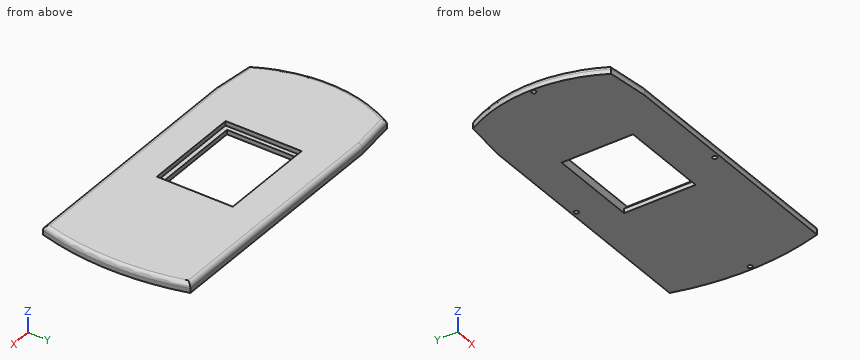
from build123d import *

# Parameters (mm, degrees)
EXTRU_MINCE1_DEPTH      = 10
ESQUISSE1_25_W          = 40
ESQUISSE1_25_H          = 136
ESQUISSE1_25_W_2        = 20
ESQUISSE1_25_H_2        = 2
ESQUISSE1_25_R          = 2.5
BOSS_EXTRU_3_DEPTH      = 10
ESQUISSE1_26_R          = 2.5
ENL_V_MAT_EXTRU_1_DEPTH = 5
ESQUISSE1_27_R          = 2.5
ENL_V_MAT_EXTRU_2_DEPTH = 5
ESQUISSE1_28_R          = 2.5
ENL_V_MAT_EXTRU_3_DEPTH = 5
ESQUISSE1_29_R          = 2.5
ENL_V_MAT_EXTRU_4_DEPTH = 5
CONG_5_R                = 5
BOSS_EXTRU_4_DEPTH      = 5


with BuildPart() as part:
    # Esquisse1 → Extru.-Mince1 (new body)
    with BuildSketch(Plane.XY):
        with BuildLine():
            Line((-199.071776485, 47.699787448), (-153.336718001, 52.844981528))
            Line((-153.336718001, 52.844981528), (122.846559315, 52.844981528))
            ThreePointArc((122.846559315, 52.844981528), (134.520037722, -29.655018472), (122.846559315, -112.155018472))
            Line((122.846559315, -112.155018472), (-153.336718001, -112.155018472))
            Line((-153.336718001, -112.155018472), (-199.071776485, -107.009824393))
            ThreePointArc((-199.071776485, -107.009824393), (-219.440219924, -29.655018472), (-199.071776485, 47.699787448))
        make_face()
        with BuildLine():
            Line((-192.775986612, 38.344981528), (-152.775986612, 42.844981528))
            Line((-152.775986612, 42.844981528), (115.224013388, 42.844981528))
            ThreePointArc((115.224013388, 42.844981528), (124.520037722, -29.655018472), (115.224013388, -102.155018472))
            Line((115.224013388, -102.155018472), (-152.775986612, -102.155018472))
            Line((-152.775986612, -102.155018472), (-192.775986612, -97.655018472))
            ThreePointArc((-192.775986612, -97.655018472), (-209.440219924, -29.655018472), (-192.775986612, 38.344981528))
        make_face(mode=Mode.SUBTRACT)
    extrude(amount=EXTRU_MINCE1_DEPTH)

    # Esquisse1_25 → Boss.-Extru.3 (add)
    # profile 1 of 14: a face of its own
    with BuildSketch(Plane.XY):
        Polygon((-192.775986612, 42.844981528), (-192.775986612, 38.344981528), (-152.775986612, 42.844981528), align=None)
    # profile 2 of 14: a face of its own
    with BuildSketch(Plane.XY):
        with Locations((-172.775986612, -29.655018472)):
            Rectangle(ESQUISSE1_25_W, ESQUISSE1_25_H)
    # profile 3 of 14: a face of its own
    with BuildSketch(Plane.XY):
        Polygon((-152.775986612, 42.844981528), (-192.775986612, 38.344981528), (-152.775986612, 38.344981528), align=None)
    # profile 4 of 14: a face of its own
    with BuildSketch(Plane.XY):
        with BuildLine():
            Line((-192.775986612, -97.655018472), (-192.775986612, 38.344981528))
            ThreePointArc((-192.775986612, 38.344981528), (-209.440219924, -29.655018472), (-192.775986612, -97.655018472))
        make_face()
    # profile 5 of 14: a face of its own
    with BuildSketch(Plane.XY):
        Polygon((-144.987389646, 42.844981528), (-152.775986612, 42.844981528), (-152.775986612, 38.344981528), (-152.775986612, -97.655018472), (-152.775986612, -102.155018472), (-144.987389646, -102.155018472), (-144.987389646, -100.155018472), (-124.987389646, -100.155018472), (-124.987389646, -102.155018472), (115.224013388, -102.155018472), (115.224013388, 42.844981528), (-124.987389646, 42.844981528), (-124.987389646, 40.844981528), (-144.987389646, 40.844981528), align=None)
        Polygon((-112.169243918, 12.844981528), (-107.169243918, 12.844981528), (-7.169243918, 12.844981528), (-2.169243918, 12.844981528), (-2.169243918, -72.155018472), (-112.169243918, -72.155018472), align=None, mode=Mode.SUBTRACT)
    # profile 6 of 14: a face of its own
    with BuildSketch(Plane.XY):
        Polygon((-152.775986612, -102.155018472), (-192.775986612, -97.655018472), (-192.775986612, -102.155018472), align=None)
    # profile 7 of 14: a face of its own
    with BuildSketch(Plane.XY):
        Polygon((-152.775986612, -97.655018472), (-192.775986612, -97.655018472), (-152.775986612, -102.155018472), align=None)
    # profile 8 of 14: a face of its own
    with BuildSketch(Plane.XY):
        with Locations((-134.987389646, 41.844981528)):
            Rectangle(ESQUISSE1_25_W_2, ESQUISSE1_25_H_2)
    # profile 9 of 14: a face of its own
    with BuildSketch(Plane.XY):
        with Locations((-134.987389646, -101.155018472)):
            Rectangle(ESQUISSE1_25_W_2, ESQUISSE1_25_H_2)
    # profile 10 of 14: a face of its own
    with BuildSketch(Plane.XY):
        with BuildLine():
            ThreePointArc((115.224013388, -102.155018472), (124.520037722, -29.655018472), (115.224013388, 42.844981528))
            Line((115.224013388, 42.844981528), (115.224013388, -102.155018472))
        make_face()
    # profile 11 of 14: a face of its own
    with BuildSketch(Plane.XY):
        with Locations((-215.775986612, -32.155018472)):
            Circle(ESQUISSE1_25_R)
    # profile 12 of 14: a face of its own
    with BuildSketch(Plane.XY):
        with Locations((130.224013388, -32.155018472)):
            Circle(ESQUISSE1_25_R)
    # profile 13 of 14: a face of its own
    with BuildSketch(Plane.XY):
        with Locations((-33.549027095, -107.155018472)):
            Circle(ESQUISSE1_25_R)
    # profile 14 of 14: a face of its own
    with BuildSketch(Plane.XY):
        with Locations((-33.549027095, 47.844981528)):
            Circle(ESQUISSE1_25_R)
    extrude(amount=BOSS_EXTRU_3_DEPTH)

    # Esquisse1_26 → Enl_v. mat.-Extru.1 (cut)
    with BuildSketch(Plane.XY):
        with Locations((130.224013388, -32.155018472)):
            Circle(ESQUISSE1_26_R)
    extrude(amount=ENL_V_MAT_EXTRU_1_DEPTH, mode=Mode.SUBTRACT)

    # Esquisse1_27 → Enl_v. mat.-Extru.2 (cut)
    with BuildSketch(Plane.XY):
        with Locations((-33.549027095, -107.155018472)):
            Circle(ESQUISSE1_27_R)
    extrude(amount=ENL_V_MAT_EXTRU_2_DEPTH, mode=Mode.SUBTRACT)

    # Esquisse1_28 → Enl_v. mat.-Extru.3 (cut)
    with BuildSketch(Plane.XY):
        with Locations((-33.549027095, 47.844981528)):
            Circle(ESQUISSE1_28_R)
    extrude(amount=ENL_V_MAT_EXTRU_3_DEPTH, mode=Mode.SUBTRACT)

    # Esquisse1_29 → Enl_v. mat.-Extru.4 (cut)
    with BuildSketch(Plane.XY):
        with Locations((-215.775986612, -32.155018472)):
            Circle(ESQUISSE1_29_R)
    extrude(amount=ENL_V_MAT_EXTRU_4_DEPTH, mode=Mode.SUBTRACT)

    # Cong_5
    cong_5_edges = [part.edges().sort_by_distance(p)[0] for p in [
        (134.520037722, -29.655018472, 10),
        (-15.245079343, 52.844981528, 10),
        (-176.204247243, 50.272384488, 10),
        (-219.440219924, -29.655018472, 10),
        (-176.204247243, -109.582421433, 10),
        (-15.245079343, -112.155018472, 10),
    ]]
    fillet(cong_5_edges, radius=CONG_5_R)

    # Esquisse1_30 → Boss.-Extru.4 (add)
    with BuildSketch(Plane.XY):
        Polygon((-7.169243918, -67.155018472), (-107.169243918, -67.155018472), (-107.169243918, 12.844981528), (-112.169243918, 12.844981528), (-112.169243918, -72.155018472), (-2.169243918, -72.155018472), (-2.169243918, 12.844981528), (-7.169243918, 12.844981528), align=None)
    extrude(amount=BOSS_EXTRU_4_DEPTH)


solid = part.part
Can you work these out from the model? Positions are in its coordinate system, mm. Round coordinates to 2 decimals unless told otherwise and drop trailing zeros. Write each loop counter-clockwise with the first axis right and the second up, starting at its lowest first coordinate (ties: lowest second). Pieces come first, ordered by that corner, then holes. Notation, with made-up numbers: M 73.25,88 L 132.25,88 A6 cw 132.25,97 Z; hole C 75,-2 d9. An arc over 180 degrees is marked long. Use a Markdown table: item, result.
Item 1: I want a section at A-A (x = -99.5). List the corners of the cut face in (y, z) for me, and give its area (3 significant figures).
Found:
| item | result |
|---|---|
| outline | M -112.16,0 L -67.16,0 L -67.16,5 L -72.16,5 L -72.16,10 L -107.16,10 A5 ccw -112.16,5 Z; M 12.84,0 L 52.84,0 L 52.84,5 A5 ccw 47.84,10 L 12.84,10 Z |
| area | 814 mm2 |
Item 2: If I drill on line 1 along Y through (x, z) = (-45, 4.25); line 2 along X through (y, z) = (-45.5, 8.75); line 3 along Y through (x, z) = (-101.5, 7.75), over which ranges is the centre line in solid material (lowest first)? Write a range as [from, to].
Found:
| item | result |
|---|---|
| line 1 | y = [-112.16, -67.16], [12.84, 52.84] |
| line 2 | x = [-216.94, -112.17], [-2.17, 132.4] |
| line 3 | y = [-111.33, -72.16], [12.84, 52.02] |
Item 3: I want a section at B-B (z = 6.75). List the corners of the cut face in (x, y) for me, and give its area (3 significant figures).
Found:
| item | result |
|---|---|
| outline | M -198.88,-106.71 L -153.32,-111.84 L 122.61,-111.84 A297.05 ccw 122.61,52.53 L -153.32,52.53 L -198.88,47.4 A156.76 ccw Z; hole M -112.17,-72.16 L -2.17,-72.16 L -2.17,12.84 L -112.17,12.84 Z |
| area | 46,600 mm2 |
Item 4: For pin 1 Ø1.5 at (x, y) = (-214.5, -31.5) entering from -Z; pin 2 Ø4 at (y, z) = (-46, 1.5) entering from -X; pin 3 Ø3 at (x, z) = (-175, 2.5) entering from -Y, each with a flat end and sliding along its axis, tell me the tip position at first contact or that it passes through.
Found:
| item | result |
|---|---|
| pin 1 | stops at z = 5 |
| pin 2 | stops at x = -218.78 |
| pin 3 | stops at y = -109.89 |
